```python
from build123d import *

# Parameters (mm, degrees)
F0_W     = 50.8
F0_H     = 76.2
F1_DEPTH = 12.7
F2_R     = 25.4
F3_R     = 25.39999
F4_W     = 50.7186688483
F4_H     = 13.4670715779
F5_DEPTH = 38.1
F6_W     = 14.5849827677
F6_H     = 12.6033662766
F7_DEPTH = 13.4680715779
F8_R     = 16.5120085349
F9_DEPTH = 38.101


# Not quite as in the source:
# - a fillet or chamfer is up to 0.001 mm smaller than in the source, because OpenCascade refuses the exact size


with BuildPart() as f1:
    # F0 (on Top) → F1 (new body)
    with BuildSketch(Plane.XY):
        Rectangle(F0_W, F0_H)
    extrude(amount=F1_DEPTH)

    # F2
    f2_edges = [f1.edges().sort_by_distance(p)[0] for p in [
        (25.4, -38.1, 6.35),
    ]]
    fillet(f2_edges, radius=F2_R)

    # F3 (radius 25.4 in the source; OpenCascade refuses exactly that, so slightly less here)
    f3_edges = [f1.edges().sort_by_distance(p)[0] for p in [
        (-25.4, -38.1, 6.35),
    ]]
    fillet(f3_edges, radius=F3_R)

    # F4 (on Top) → F5 (join)
    with BuildSketch(Plane.XY):
        with Locations((-0.1172143966, 31.366464211)):
            Rectangle(F4_W, F4_H)
    extrude(amount=F5_DEPTH)

    # F6 (on face) → F7 (cut, through all)
    with BuildSketch(Plane.XZ.offset(-24.6329284221)):
        with Locations((-18.1840574369, 31.7983168617)):
            Rectangle(F6_W, F6_H)
    extrude(amount=-F7_DEPTH, mode=Mode.SUBTRACT)

    # F8 (on Top) → F9 (cut, through all)
    with BuildSketch(Plane.XY):
        with Locations((0, -15.7830994576)):
            Circle(F8_R)
    extrude(amount=F9_DEPTH, mode=Mode.SUBTRACT)


solid = f1.part
```
Could you check a few things on this model? Use its own coordinates, in mm. A direction names the side the tool comes from. Give positions to 0.01 mm unless a question says otherwise; leave off trailing zeros. Write each loop counter-clockwise with the first axis right and the second up, starting at its lowest first coordinate (ties: lowest second). Pieces come first, ordered by that corner, then holes. Notation, with made-up numbers: (40.25, 15) - (95.25, 15) arc R15 cw to (95.25, 43) - close; hole circle Ø4 at (-8.75, 83). An arc over 180 degrees is marked (long way). One line per item, written item: value. Start each with the question number.
Item 1: Imagine slicing it at B-B, the plane x = 1. List the corners of the cut face in (y, z) for me, and give its area (3 significant figures).
Item 2: I'm going to push flat-ended pins straight in: pin 1 (14 mm diameter, centred on y = 9.5, z = 9, fed in from -X); pin 2 (5 mm diameter, centred on x = -20, z = 25, fed in from -Y); pin 3 (6 mm diameter, centred on x = 4, y = -26.5, fed in from +Z); pin 4 (1.5 mm diameter, centred on x = -20.5, y = 23, fed in from +Z). Where does each tip first touch, or does it pass through?
Item 3: Please list where these lines run through material, in increasing order: line 1 (Z direction, x = 0, y = -33); line 2 (Y direction, x = 21.5, z = 13); line 3 (X direction, y = 3, z = 12). Write a range as from..to.
Item 4: Which directions (+Z, -Z, +X, -X, +Y, -Y) give clear straight access to the entire face, cutting with the end or side of a thin tool? Please do faces 5 (the face through (-25.4, 6, 6)), 6 (the face through (-18, 31, 25.497)), 7 (the face through (25.242, 31, 25)).
Item 5: Imagine slicing it at D-D, the plane y = 30.5. List the corners of the cut face in (x, z) for me, and give its area (3 significant figures).
Item 6: Imagine slicing it at A-A, the plane y = -24.5. List the corners of the cut face in (x, z) for me, and give its area (3 significant figures).
Item 7: If we mould it in two halves opening along X, with no side actions, what happens to faces 1 (the face through (17.76, -30.86, 6.44)), 2 (the face through (-10.892, 31, 32)), 3 (the face through (-3.579, -31.902, 6.261)), 4 (the face through (0, 38.1, 19))? For each: +X half, -X half, draft (parallel to the pull), parting line (faces both ways), or undercut.
Geometry says:
1. outline: (-38.08, 0) - (-32.26, 0) - (-32.26, 12.7) - (-38.08, 12.7) - close; (0.7, 0) - (38.1, 0) - (38.1, 38.1) - (24.63, 38.1) - (24.63, 12.7) - (0.7, 12.7) - close
1. area: 891 mm^2
2. pin 1: x = -25.4
2. pin 2: y = 24.63
2. pin 3: through
2. pin 4: z = 12.7
3. line 1: 0..12.7
3. line 2: 24.63..38.1
3. line 3: -25.4..25.4
4. face 5: +Z, -Z, -X, -Y
4. face 6: +Z, -X, +Y, -Y
4. face 7: +Z, +X, +Y, -Y
5. outline: (-25.48, 0) - (25.4, 0) - (25.4, 12.7) - (25.24, 12.7) - (25.24, 38.1) - (-10.89, 38.1) - (-10.89, 25.5) - (-25.48, 25.5) - close
5. area: 1,750 mm^2
6. outline: (-22.49, 0) - (-14.02, 0) - (-14.02, 12.7) - (-22.49, 12.7) - close; (14.02, 0) - (22.49, 0) - (22.49, 12.7) - (14.02, 12.7) - close
6. area: 215 mm^2
7. face 1: +X half
7. face 2: -X half
7. face 3: undercut
7. face 4: draft
